The listing builds one solid part. Answer for the finished solid, in the listing's coordinates (mm). Face numbers are marked on the shaded views. Coordinates: 2 decimals unless noted, no trailing zeros. Order: outer loops, then holes, each group sorted by start corner. A loop starts at its lowest first (then second) coordinate and runs counter-clockwise, first axis right, second up. Notation, with made-up numbers: (31.5, -25.5) - (74.5, -25.5) arc R17 ccw to (74.5, -20.5) - close; hole circle Ø6 at (53, -21.75). An arc over 180 degrees is marked (long way). Use one line per item in the form item = value. Start each with the question number.
Item 1: Section B-B, the plane x = 106 is taken. Write down the section's boundary in (y, z).
Item 2: Consider line 1 along Z through (x, y) = (14, 3); line 2 along X through (y, z) = (6, 590); line 3 along Y through (x, z) = (4.5, 99.5). Determine where each line is inside the solid, lowest interval first. Write a range as [from, to].
Item 3: The mould has two halves that part along X. Classify the marked faces 1 and 2: released by +X, released by -X, zero draft, split by the parting line, or undercut.
Item 4: Section A-A, the plane z = 1155 is taken. Write down the section's boundary in (x, y), and give its area (3 significant figures).
from build123d import *

# Parameters (mm, degrees)
F0_W     = 558.8
F0_H     = 1981.2
F1_DEPTH = 19.05
F2_W     = 393.7
F2_H     = 863.6
F3_DEPTH = 6.35


with BuildPart() as f1:
    # F0 (on Front) → F1 (new body)
    with BuildSketch(Plane.XZ):
        with Locations((1.273108, 439.16639)):
            Rectangle(F0_W, F0_H)
    extrude(amount=-F1_DEPTH)

    # F2 (on face) → F3 (cut)
    with BuildSketch(Plane.XZ):
        with Locations((1.273108, 915.41639)):
            Rectangle(F2_W, F2_H)
        with Locations((1.273108, -37.08361)):
            Rectangle(F2_W, F2_H)
    extrude(amount=-F3_DEPTH, mode=Mode.SUBTRACT)


solid = f1.part
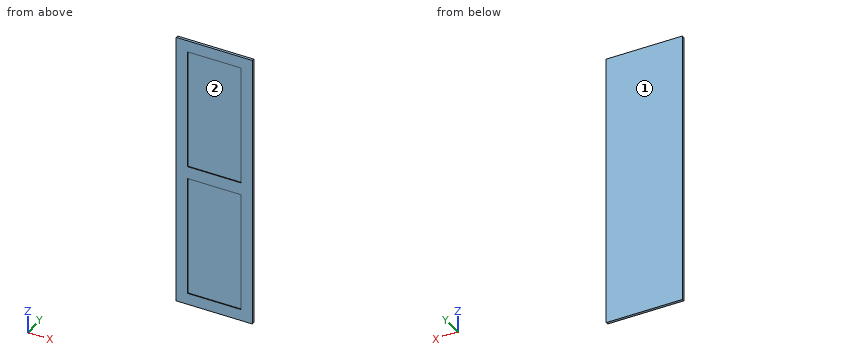
Response:
q1.outline = (0, -551.43) - (19.05, -551.43) - (19.05, 1429.77) - (0, 1429.77) - (0, 1347.22) - (6.35, 1347.22) - (6.35, 483.62) - (0, 483.62) - (0, 394.72) - (6.35, 394.72) - (6.35, -468.88) - (0, -468.88) - close
q2.line_1 = [-551.43, -468.88], [394.72, 483.62], [1347.22, 1429.77]
q2.line_2 = [-278.13, -195.58], [198.12, 280.67]
q2.line_3 = [6.35, 19.05]
q3.face_1 = zero draft
q3.face_2 = undercut
q4.outline = (-278.13, 0) - (-195.58, 0) - (-195.58, 6.35) - (198.12, 6.35) - (198.12, 0) - (280.67, 0) - (280.67, 19.05) - (-278.13, 19.05) - close
q4.area = 8,150 mm2
